```python
from build123d import *

# Parameters (mm, degrees)
CROQUIS1_R              = 3.175
SALIENTE_EXTRUIR1_DEPTH = 25
REDONDEO1_R             = 10
CORTAR_EXTRUIR1_DEPTH   = 16
REDONDEO2_R             = 5


with BuildPart() as part:
    # Croquis1 → Saliente-Extruir1 (new body, symmetric)
    with BuildSketch(Plane.XY):
        with BuildLine():
            Line((-4, 17.843284464), (-11.233642387, 21.995392823))
            ThreePointArc((-11.233642387, 21.995392823), (-11.258169907, 34.990466775), (0, 28.5))
            Line((0, 28.5), (0, -28.5))
            ThreePointArc((0, -28.5), (-11.258169907, -34.990466775), (-11.233642387, -21.995392823))
            Line((-11.233642387, -21.995392823), (-4, -17.843284464))
            Line((-4, -17.843284464), (-4, 17.843284464))
        make_face()
        with Locations((-7.5, 28.5)):
            Circle(CROQUIS1_R, mode=Mode.SUBTRACT)
        with Locations((-7.5, -28.5)):
            Circle(CROQUIS1_R, mode=Mode.SUBTRACT)
    extrude(amount=SALIENTE_EXTRUIR1_DEPTH, both=True)

    # Redondeo1
    redondeo1_edges = [part.edges().sort_by_distance(p)[0] for p in [
        (-4, -17.843284464, 0),
        (-4, 17.843284464, 0),
    ]]
    fillet(redondeo1_edges, radius=REDONDEO1_R)

    # Croquis2 → Cortar-Extruir1 (cut, through all)
    with BuildSketch(Plane(origin=(0, 0, 0), x_dir=(0, 0, -1), z_dir=(1, 0, 0))):
        Polygon((-9, 25), (-5, 12.159257653), (-5, -12.159257653), (-9, -25), (-29.873538988, -25), (-29.873538988, 25), align=None)
    extrude(amount=-CORTAR_EXTRUIR1_DEPTH, mode=Mode.SUBTRACT)

    # Redondeo2
    redondeo2_edges = [part.edges().sort_by_distance(p)[0] for p in [
        (-2.000282316, 12.159257653, 5),
        (-2.000282316, -12.159257653, 5),
        (-7.06662479, -25, 9),
        (-7.06662479, 25, 9),
    ]]
    fillet(redondeo2_edges, radius=REDONDEO2_R)


solid = part.part
```
The listing builds one solid part. Answer for the finished solid, in the listing's coordinates (mm). A direction names the side the tool comes from. Give positions to 0.01 mm unless a question says otherwise; leave off trailing zeros. Loops run counter-clockwise (first coordinate to the right, second up) from the corner with the lowest first, then second, coordinate; pieces in that order, holes last. Notation, with made-up numbers: (-24.5, -14.5) - (-5.5, -14.5) arc R19 ccw to (-5.5, 2.5) - close; hole circle Ø1 at (29.25, 60). An arc over 180 degrees is marked (long way). Answer as CSV lines item,"result". Start each with the question number.
Item 1: A cutting plane is placed at B-B on x = -7.5. Determine the outline of the cut face in (y, z) (3 decimals), then the cut area to 3 significant figures.
Item 2: A cutting plane is placed at D-D on y = -1. Determine the outline of the cut face in (x, z).
Item 3: Each of these flat-tipped pins is pushed along its axis until it touches: pin 1 (1.2 mm diameter, centred on x = -2.5, y = -5.5, fed in from +Z); pin 2 (6 mm diameter, centred on x = -3.5, z = 11.5, fed in from +Y); pin 3 (3.5 mm diameter, centred on x = -10, z = 20, fed in from -Y). Where does it stop, or does it pass through?
Item 4: The mould has two halves that part along X. Classify faces 4 (the face through (-8.19, -31.6, -0.35)), 5 (the face through (-11.066, -35.098, 0.35)), 6 (the face through (-7, -25, 19)), 7 (the face through (-10.11, 21.35, -8.22)): +X half, -X half, draft (parallel to the pull), parting line (faces both ways), or undercut.
Item 5: A cutting plane is placed at A-A on z = 14.5. Determine the outline of the cut face in (x, y) (3 decimals), then the cut area to 3 significant figures.
Item 6: A cutting plane is placed at C-C on z = -6. Determine the outline of the cut face in (x, y) (3 decimals), then the cut area to 3 significant figures.
Item 7: Find the intervals of material crossed by line 1 (Y direction, x = -7.5, z = 14.5) (3 decimals); line 2 (Y direction, x = -7.5, z = -10) (3 decimals); line 3 (X direction, y = 10.5, z = -10), in increasing order. Write a range as from..to.
Item 8: For faces 1 (the face through (-4, 0, -10)), 2 (the face through (-2.8, 18.2, 6.88)), 3 (the face through (-2, 1, -25)), determine the directions among +Z, -Z, +X, -X, +Y, -Y from which every point of the face is accessible in a straight line to the end or side of a thin tool.
Found:
1,outline,"(-36, -25) - (-31.675, -25) - (-31.675, 25) - (-36, 25) - close; (-25.325, -25) - (-19.652, -25) - (-19.652, 7.334) - (-21.487, 7.906) arc R5 cw to (-25, 12.679) - (-25, 25) - (-25.325, 25) - close; (19.652, -25) - (25.325, -25) - (25.325, 25) - (25, 25) - (25, 12.679) arc R5 cw to (21.487, 7.906) - (19.652, 7.334) - close; (31.675, -25) - (36, -25) - (36, 25) - (31.675, 25) - close"
1,area,"825 mm^2"
2,outline,"(-4, -25) - (0, -25) - (0, 5) - (-4, 5) - close"
3,pin 1,"stops at z = 5"
3,pin 2,"stops at y = 35.93"
3,pin 3,"stops at y = -35.96"
4,face 4,"undercut"
4,face 5,"parting line"
4,face 6,"draft"
4,face 7,"-X half"
5,outline,"(-14.133, -25) arc R7.5 ccw (long way) to (0, -28.5) - (0, -25) - close; (-14.133, 25) - (0, 25) - (0, 28.5) arc R7.5 ccw (long way) to start; hole circle Ø6.35 at (-7.5, -28.5); hole circle Ø6.35 at (-7.5, 28.5)"
5,area,"216 mm^2"
6,outline,"(-11.234, -21.995) arc R7.5 ccw (long way) to (0, -28.5) - (0, 28.5) arc R7.5 ccw (long way) to (-11.234, 21.995) - (-9.022, 20.726) arc R10 cw to (-4, 12.053) - (-4, -12.053) arc R10 cw to (-9.022, -20.726) - close; hole circle Ø6.35 at (-7.5, -28.5); hole circle Ø6.35 at (-7.5, 28.5)"
6,area,"511 mm^2"
7,line 1,"y = -36..-31.675, -25.325..-25, 25..25.325, 31.675..36"
7,line 2,"y = -36..-31.675, -25.325..-19.652, 19.652..25.325, 31.675..36"
7,line 3,"x = -4..0"
8,face 1,"+Z, -Z, -X"
8,face 2,"+Z, +X, -X"
8,face 3,"-Z, +X, -X, +Y, -Y"
